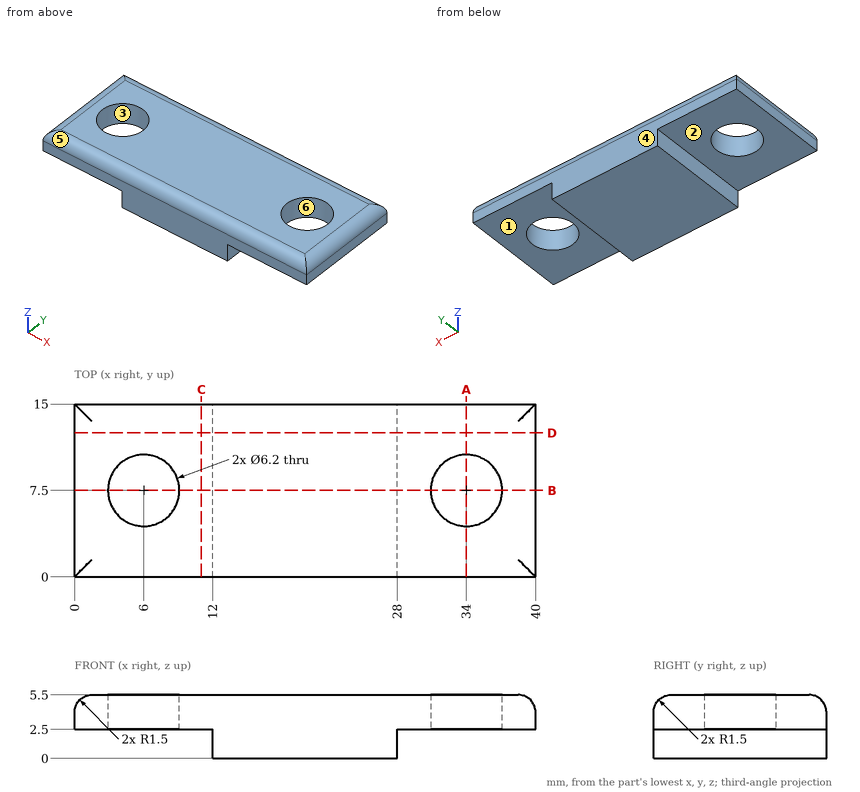
Input: dimensioned drawing with shaded views. Units: mm. Origin: part minimum x, y, z. A direction names the side the tool comes from. Coordinates: 2 decimals unless noted, no trailing zeros. Loops run counter-clockwise (first coordinate to the right, second up) from the corner with the lowest first, then second, coordinate; pieces in that order, holes last. Notation, with made-up numbers: M 13.25,-31.75 L 34.25,-31.75 A17 ccw 34.25,-6.75 Z; hole C 30.25,56 d8. An arc over 180 degrees is marked long. Put each result on its own line as item: value.
(1) First-contact query: pin 1 (2 mm diameter, centred on y = 9, z = 1, fed in from +X); pin 2 (5 mm diameter, centred on x = 13, y = 2.5, fed in from -Z); pin 3 (3.5 mm diameter, centred on x = 35, y = 8, fed in from -Z); pin 4 (8 mm diameter, centred on x = 34, y = 7.5, fed in from -Z). Flat tips, straight axial feed; report the tip coordinate or a pass-through.
Answer sheet:
pin 1: stops at x = 28
pin 2: stops at z = 0
pin 3: passes through
pin 4: stops at z = 2.5
(2) Cut plane A-A on x = 34. Return the cut outline in (y, z), then the cut area to 3 significant figures.
Answer sheet:
outline: M 0,2.5 L 4.4,2.5 L 4.4,5.5 L 1.5,5.5 A1.5 ccw 0,4 Z; M 10.6,2.5 L 15,2.5 L 15,4 A1.5 ccw 13.5,5.5 L 10.6,5.5 Z
area: 25.4 mm^2
(3) Draft query along Y for the marked faces 4, 5 and 6. Return one class per face: pulls with the +Y half, pulls with the -Y half, needs draft (parallel to the pull), parting line crosses it, or undercut.
Answer sheet:
face 4: pulls with the +Y half
face 5: pulls with the -Y half
face 6: undercut
(4) Cut plane C-C on x = 11. Return the cut outline in (y, z).
Answer sheet:
outline: M 0,2.5 L 15,2.5 L 15,4 A1.5 ccw 13.5,5.5 L 1.5,5.5 A1.5 ccw 0,4 Z
(5) Material intervals for probe 1 along Y at (x, z) = (6, 2.85); probe 2 along X at (y, z) = (8.25, 4.5); probe 3 along X at (y, z) = (6, 5.1), sorted ascending.
Answer sheet:
probe 1: y = 0 to 4.4, 10.6 to 15
probe 2: x = 0.09 to 2.99, 9.01 to 30.99, 37.01 to 39.91
probe 3: x = 0.48 to 3.29, 8.71 to 31.29, 36.71 to 39.52
(6) Access query for the marked faces 1, 2 and 3. Directions: +Z, -Z, +X, -X, +Y, -Y. A direction counts if a zero-diameter tool reaches every point of the face in a straight line with its end or side. Return the directions, or none.
Answer sheet:
face 1: -Z, +X, +Y, -Y
face 2: -Z, -X, +Y, -Y
face 3: +Z, -Z
(7) Cut plane D-D on y = 12.5. Return the cut outline in (x, z), then the cut area to 3 significant figures.
Answer sheet:
outline: M 0,2.5 L 12,2.5 L 12,0 L 28,0 L 28,2.5 L 40,2.5 L 40,4 A1.5 ccw 38.5,5.5 L 1.5,5.5 A1.5 ccw 0,4 Z
area: 159 mm^2
(8) Cut plane B-B on y = 7.5. Return the cut outline in (x, z).
Answer sheet:
outline: M 0,2.5 L 2.9,2.5 L 2.9,5.5 L 1.5,5.5 A1.5 ccw 0,4 Z; M 9.1,2.5 L 12,2.5 L 12,0 L 28,0 L 28,2.5 L 30.9,2.5 L 30.9,5.5 L 9.1,5.5 Z; M 37.1,2.5 L 40,2.5 L 40,4 A1.5 ccw 38.5,5.5 L 37.1,5.5 Z
